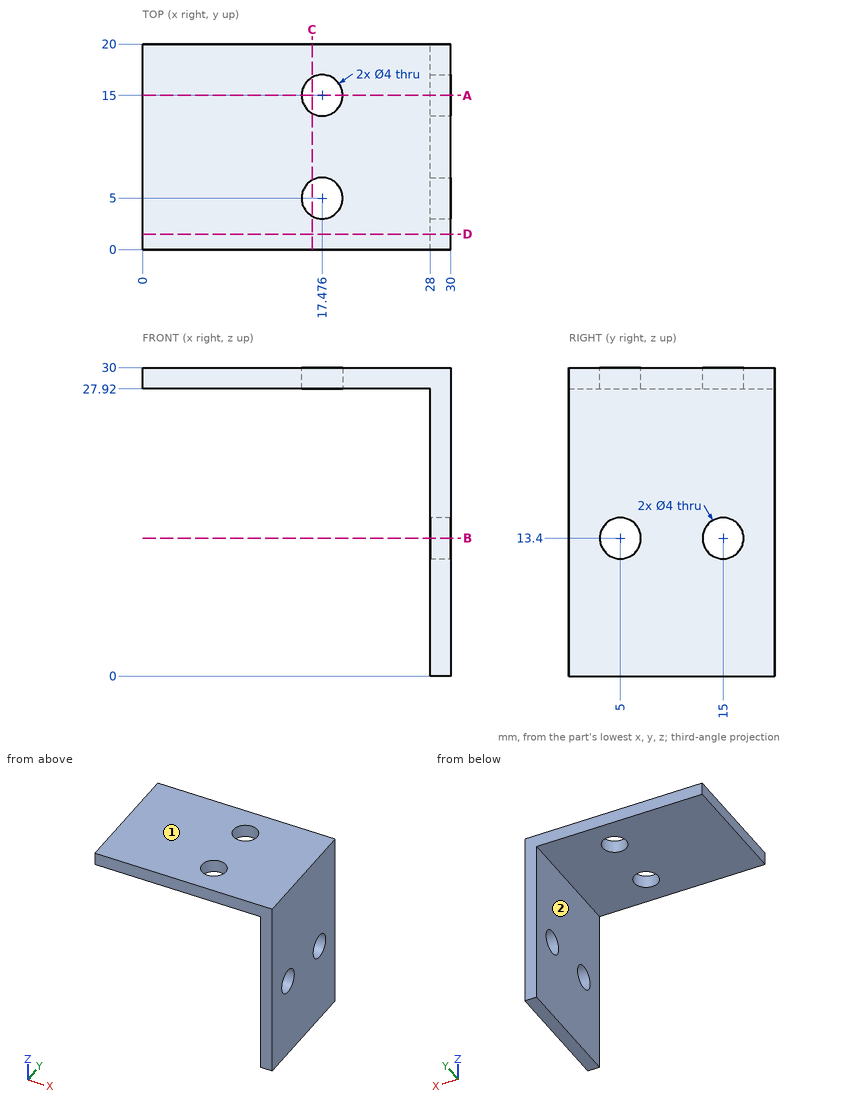
Geometry: see drawing. Coordinates: mm, zero at the bounding-box minimum. A direction names the side the tool comes from. Round coordinates to 2 decimals unless told otherwise and drop trailing zeros. Write each loop counter-clockwise with the first axis right and the second up, starting at its lowest first coordinate (ties: lowest second). Pieces come first, ordered by that corner, then holes.
1) Cut plane A-A (y = 15). Return the cut outline in (x, z).
2) Cut plane C-C (x = 16.5). Return the cut outline in (y, z).
3) Ray query, L1, parallel to Y at x = 28.5, z = 13.4; L2, parallel to X at y = 7.5, z = 21.5; L3, parallel to Z at x = 10.5, y = 7.75. Return the intervals inside material, ascending.
4) Cut plane B-B (z = 13.4). Return the cut outline in (x, y), then the cut area to 3 significant figures.
5) Reachability of the marked faces 1 and 2 from +Z, -Z, +X, -X, +Y, -Y: full face, straight path, thin tool, end or side. Return the list, or none.
6) Cut plane D-D (y = 1.5). Return the cut outline in (x, z).
7) Contact query for flat-ended pins moving along their axis: P1, Ø5, axis at x = 17.48, y = 5, coming from the +Z side; P2, Ø6, axis at y = 5, z = 16, coming from the -X side; P3, Ø6, axis at x = 9.5, y = 11, coming from the -Z side; P4, Ø3, axis at y = 5, z = 13.4, coming from the +X side. Output: stop coordinate, or through.
Geometry says:
1. outline: (0, 27.92) - (15.48, 27.92) - (15.48, 30) - (0, 30) - close; (19.48, 27.92) - (28, 27.92) - (28, 15.4) - (30, 15.4) - (30, 30) - (19.48, 30) - close; (28, 0) - (30, 0) - (30, 11.4) - (28, 11.4) - close
2. outline: (0, 27.92) - (3.25, 27.92) - (3.25, 30) - (0, 30) - close; (6.75, 27.92) - (13.25, 27.92) - (13.25, 30) - (6.75, 30) - close; (16.75, 27.92) - (20, 27.92) - (20, 30) - (16.75, 30) - close
3. L1: y = 0 to 3, 7 to 13, 17 to 20
3. L2: x = 28 to 30
3. L3: z = 27.92 to 30
4. outline: (28, 0) - (30, 0) - (30, 3) - (28, 3) - close; (28, 7) - (30, 7) - (30, 13) - (28, 13) - close; (28, 17) - (30, 17) - (30, 20) - (28, 20) - close
4. area: 24.0 mm2
5. face 1: +Z, +X, -X, +Y, -Y
5. face 2: -Z, -X, +Y, -Y
6. outline: (0, 27.92) - (28, 27.92) - (28, 0) - (30, 0) - (30, 30) - (0, 30) - close
7. P1: stops at z = 30
7. P2: stops at x = 28
7. P3: stops at z = 27.92
7. P4: passes through
